The listing builds one solid part. Answer for the finished solid, in the listing's coordinates (mm). Face numbers are marked on the shaded views. A direction names the side the tool comes from. Round coordinates to 2 decimals unless told otherwise and drop trailing zeros. Loops run counter-clockwise (first coordinate to the right, second up) from the corner with the lowest first, then second, coordinate; pieces in that order, holes last. Notation, with made-up numbers: M -29,45.5 L -14,45.5 A17 cw -14,65.5 Z; hole C -19.5,64 d4. An arc over 180 degrees is marked long. Answer as a JSON object with one key per item and string values.
```python
from build123d import *

# Parameters (mm, degrees)
BOSS_EXTRUDE1_DEPTH = 16.51
CUT_EXTRUDE1_DEPTH  = 50.74516387
SKETCH4_R           = 1.5875
CUT_EXTRUDE2_DEPTH  = 54.238681437
BOSS_EXTRUDE3_DEPTH = 1.27
BOSS_EXTRUDE4_DEPTH = 1.27
SKETCH11_W          = 10.16
SKETCH11_H          = 7.62
BOSS_EXTRUDE5_DEPTH = 2.54
BOSS_EXTRUDE5_TAPER = 4
SKETCH12_R          = 1.5875
CUT_EXTRUDE3_DEPTH  = 63.462199051
CUT_EXTRUDE4_DEPTH  = 3.302
FILLET1_R           = 0.762
SKETCH14_R          = 1.5875
CUT_EXTRUDE6_DEPTH  = 65.202975796
CUT_EXTRUDE7_DEPTH  = 3.302
CUT_EXTRUDE10_DEPTH = 76.2


with BuildPart() as part:
    # Sketch1 → Boss-Extrude1 (new body)
    with BuildSketch(Plane(origin=(0, 0, 0), x_dir=(1, 0, 0), z_dir=(0, 1, 0))):
        with BuildLine():
            Line((-7.62, -31.114876642), (-7.62, -40.004876642))
            ThreePointArc((-7.62, -40.004876642), (-6.876051224, -41.800927866), (-5.08, -42.544876642))
            Line((-5.08, -42.544876642), (5.08, -42.544876642))
            ThreePointArc((5.08, -42.544876642), (6.876051224, -41.800927866), (7.62, -40.004876642))
            Line((7.62, -40.004876642), (7.62, -31.114876642))
            Line((7.62, -31.114876642), (19.797340731, -24.084285693))
            Line((19.797340731, -24.084285693), (19.797340731, -1.224285693))
            Line((19.797340731, -1.224285693), (0, 10.205714307))
            Line((0, 10.205714307), (-19.797340731, -1.224285693))
            Line((-19.797340731, -1.224285693), (-19.797340731, -24.084285693))
            Line((-19.797340731, -24.084285693), (-7.62, -31.114876642))
        make_face()
        Polygon((0, 9.189714307), (-18.91745892, -1.732285693), (-18.91745892, -23.576285693), (0, -34.498285693), (18.91745892, -23.576285693), (18.91745892, -1.732285693), align=None, mode=Mode.SUBTRACT)
    extrude(amount=BOSS_EXTRUDE1_DEPTH)

    # Sketch2 → Cut-Extrude1 (cut, through all)
    with BuildSketch(Plane(origin=(0, 16.51, 0), x_dir=(1, 0, 0), z_dir=(0, 1, 0))):
        Polygon((-0.762, -34.058344788), (-0.762, -42.544876642), (0.762, -42.544876642), (0.762, -34.058344788), (0, -34.498285693), align=None)
    extrude(amount=-CUT_EXTRUDE1_DEPTH, mode=Mode.SUBTRACT)

    # Sketch4 → Cut-Extrude2 (cut, through all)
    with BuildSketch(Plane.ZY.offset(7.62)):
        with Locations((35.559876642, 8.255)):
            Circle(SKETCH4_R)
    extrude(amount=-CUT_EXTRUDE2_DEPTH, mode=Mode.SUBTRACT)

    # Sketch8 → Boss-Extrude3 (add)
    with BuildSketch(Plane(origin=(0, 16.51, 0), x_dir=(1, 0, 0), z_dir=(0, 1, 0))):
        Polygon((-10.419364221, -7.085804169), (10.419364221, -7.085804169), (18.91745892, -12.654285693), (19.797340731, -12.654285693), (19.797340731, -1.224285693), (0, 10.205714307), (-19.797340731, -1.224285693), (-19.797340731, -12.654285693), (-18.91745892, -12.654285693), align=None)
    extrude(amount=BOSS_EXTRUDE3_DEPTH)

    # Sketch9 → Boss-Extrude4 (add)
    with BuildSketch(Plane.XZ):
        Polygon((-10.419364221, 7.085804169), (10.419364221, 7.085804169), (18.91745892, 12.654285693), (19.797340731, 12.654285693), (19.797340731, 1.224285693), (0, -10.205714307), (-19.797340731, 1.224285693), (-19.797340731, 12.654285693), (-18.91745892, 12.654285693), align=None)
    extrude(amount=BOSS_EXTRUDE4_DEPTH)

    # Sketch11 → Boss-Extrude5 (add)
    with BuildSketch(Plane.ZY.offset(19.797340731)):
        with Locations((10.114285693, 9.525)):
            Rectangle(SKETCH11_W, SKETCH11_H)
    boss_extrude5 = extrude(amount=BOSS_EXTRUDE5_DEPTH, taper=BOSS_EXTRUDE5_TAPER)

    # Sketch12 → Cut-Extrude3 (cut, through all)
    with BuildSketch(Plane.ZY.offset(22.337340731)):
        with Locations((10.114285693, 9.525)):
            Circle(SKETCH12_R)
    extrude(amount=-CUT_EXTRUDE3_DEPTH, mode=Mode.SUBTRACT)

    # Sketch13 → Cut-Extrude4 (cut)
    with BuildSketch(Plane(origin=(-18.91745892, 0, 0), x_dir=(0, 0, -1), z_dir=(1, 0, 0))):
        Polygon((-8.336285693, 12.604586336), (-11.892285693, 12.604586336), (-13.670285693, 9.525), (-11.892285693, 6.445413664), (-8.336285693, 6.445413664), (-6.558285693, 9.525), align=None)
    cut_extrude4 = extrude(amount=-CUT_EXTRUDE4_DEPTH, mode=Mode.SUBTRACT)

    # Mirror1: Boss-Extrude5, Cut-Extrude4 across plane
    add(boss_extrude5.mirror(Plane(origin=(0, 0, 0), x_dir=(0, 0, 1), z_dir=(1, 0, 0))))
    add(cut_extrude4.mirror(Plane(origin=(0, 0, 0), x_dir=(0, 0, 1), z_dir=(1, 0, 0))), mode=Mode.SUBTRACT)

    # Fillet1
    fillet1_edges = [part.edges().sort_by_distance(p)[0] for p in [
        (18.91745892, 8.255, 1.732285693),
        (0, 8.255, -9.189714307),
        (-18.91745892, 8.255, 1.732285693),
        (-18.91745892, 8.255, 23.576285693),
        (18.91745892, 8.255, 23.576285693),
    ]]
    fillet(fillet1_edges, radius=FILLET1_R)

    # Sketch14 → Cut-Extrude6 (cut, through all)
    with BuildSketch(Plane(origin=(22.337340731, 0, 0), x_dir=(0, 0, -1), z_dir=(1, 0, 0))):
        with Locations(Location((-10.114285693, 9.525, 0), (0, 0, 180))):
            Circle(SKETCH14_R)
    extrude(amount=-CUT_EXTRUDE6_DEPTH, mode=Mode.SUBTRACT)

    # Sketch15 → Cut-Extrude7 (cut)
    with BuildSketch(Plane.ZY.offset(7.62)):
        Polygon((35.559876642, 11.811), (32.480290306, 10.033), (32.480290306, 6.477), (35.559876642, 4.699), (38.639462978, 6.477), (38.639462978, 10.033), align=None)
    extrude(amount=-CUT_EXTRUDE7_DEPTH, mode=Mode.SUBTRACT)

    # Sketch16 → Cut-Extrude10 (cut)
    with BuildSketch(Plane(origin=(0, 17.78, 0), x_dir=(1, 0, 0), z_dir=(0, 1, 0))):
        with BuildLine():
            Line((-6.260612009, -7.085804169), (6.260612009, -7.085804169))
            ThreePointArc((6.260612009, -7.085804169), (0, -1.797518476), (-6.260612009, -7.085804169))
        make_face()
    extrude(amount=-CUT_EXTRUDE10_DEPTH, mode=Mode.SUBTRACT)


solid = part.part
```
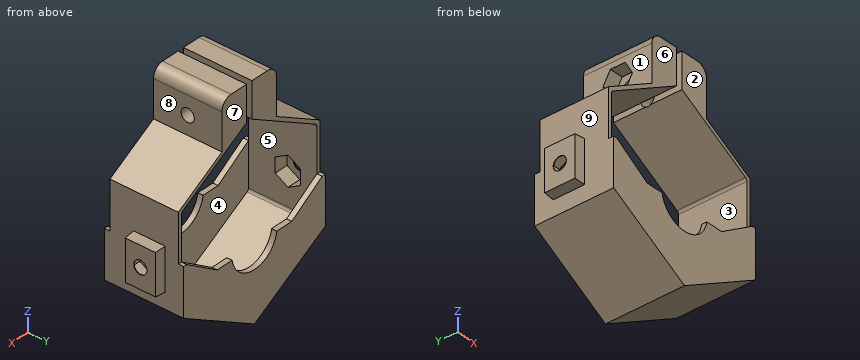
Item 1: Flat-ended cylindrical pins translate along their axes: P1, Ø1.7, axis at x = -21.5, z = 10, coming from the -Y side; P2, Ø21, axis at x = -6.5, z = 34, coming from the +Y side; P3, Ø7, axis at y = 10, z = 40, coming from the -X side. Find the tip coordinate at first contact, or state that the pin passes through.
Values follow:
{"P1": "y = 5.77", "P2": "y = 16.51", "P3": "x = -7.62"}
Item 2: The part is cut by section A-A (z = 21). Give the vertices of the cut face in (x, y).
Values follow:
{"outline": "M -19.8,0 L -18.92,0 L -18.92,16.51 L -19.8,16.51 Z; M 18.92,0 L 19.8,0 L 19.8,16.51 L 18.92,16.51 Z"}
Item 3: The part is cut by section C-C (x = 11). Give the vertices of the cut face in (y, z), then the cut area to 3 significant figures.
Values follow:
{"outline": "M -1.27,-3.85 L 17.78,-3.85 L 17.78,7.47 L 16.51,7.47 L 16.51,-2.84 L 0,-2.84 L 0,7.47 L -1.27,7.47 Z; M 0,28.15 L 16.51,28.15 L 16.51,29.16 L 0,29.16 Z", "area": "62.3 mm^2"}
Item 4: Straight lines are drawn through the part: line 1 (X direction, y = 2.5, z = 39.5); line 2 (Y direction, x = -9, z = -3); line 3 (X direction, y = 5, z = 4.5). For each, find the intervals that lie inside material, in ascending order.
Values follow:
{"line 1": "-7.62 to -0.76, 0.76 to 7.62", "line 2": "-1.27 to 0, 16.51 to 17.78", "line 3": "-19.8 to -18.92, 18.92 to 19.8"}
Item 5: The part is cut by section B-B (y = 2.5). Give the vertices of the cut face in (x, z).
Values follow:
{"outline": "M -19.8,1.22 L 0,-10.21 L 19.8,1.22 L 19.8,24.08 L 7.62,31.11 L 7.62,40 A2.54 ccw 5.08,42.54 L 0.76,42.54 L 0.76,34.06 L 18.54,23.8 A0.76 cw 18.92,23.14 L 18.92,2.17 A0.76 cw 18.54,1.51 L 0.38,-8.97 A0.76 cw -0.38,-8.97 L -18.54,1.51 A0.76 cw -18.92,2.17 L -18.92,23.14 A0.76 cw -18.54,23.8 L -0.76,34.06 L -0.76,42.54 L -5.08,42.54 A2.54 ccw -7.62,40 L -7.62,31.11 L -19.8,24.08 Z"}
Item 6: Which of the six approach directions +Z, -Z, +X, -X, +Y, -Y give full straight-line access (tool end or side, diameter ignored) to the marked faces 5, 6, 7, 8 and 9?
Values follow:
{"face 5": "none", "face 6": "+Z, +X, -X, -Y", "face 7": "+Z, +X, -X, +Y", "face 8": "+Z, +X, +Y, -Y", "face 9": "-X"}
Item 7: The part is cut by section D-D (z = 38). Give the vertices of the cut face in (x, y), then the cut area to 3 significant figures.
Values follow:
{"outline": "M -7.62,0 L -0.76,0 L -0.76,16.51 L -7.62,16.51 L -7.62,10.4 L -4.32,10.4 L -4.32,6.11 L -7.62,6.11 Z; M 0.76,0 L 7.62,0 L 7.62,16.51 L 0.76,16.51 Z", "area": "212 mm^2"}
Item 8: Determine the mould class of the marked faces 1, 2, 3 and 4 for opening direction Y: released by +Y, released by -Y, zero draft, split by the parting line, or undercut.
Values follow:
{"face 1": "zero draft", "face 2": "released by -Y", "face 3": "undercut", "face 4": "undercut"}
